Read the model definition and answer for the solid it produces. Units are mm, in the model's axes. Face numbers are marked on the shaded views. A direction names the side the tool comes from. Coordinates: 2 decimals unless noted, no trailing zeros. Order: outer loops, then holes, each group sorted by start corner. A loop starts at its lowest first (then second) coordinate and runs counter-clockwise, first axis right, second up. Notation, with made-up numbers: (-22, -36.5) -> (24, -36.5) arc R18 ccw to (24, -25.5) -> close; hole circle Ø2 at (69, 44). An arc over 180 degrees is marked (long way). Answer as a JSON object with one key per item and string values. Group by question number.
1) Given pin 1 (4 mm diameter, centred on x = 0.5, z = 7, fed in from -Y); pin 2 (1.4 mm diameter, centred on x = 1, z = -7, fed in from +Y); pin 3 (2.5 mm diameter, centred on y = 0, z = 12, fed in from -X), each flat-ended and moving along its own axis, determine where each tip first touches the part or whether it passes through.
2) Section C-C on z = 12 is taken. Count the separate pieces of the cut face and the enclosed holes in it, and give its area (3 significant figures).
3) Section B-B on y = 1.25 is taken. Determine the outline of the cut face in (x, z), and give its area (3 significant figures).
4) Consider L1, parallel to X at y = -8, z = 23.5; L2, parallel to Y at x = -3, z = 9; L3, parallel to Y at x = -4, z = 16. Determine where each line is inside the solid, lowest interval first.
5) Section A-A on x = -6 is taken. Determine the outline of the cut face in (y, z), and give its area (3 significant figures).
6) Determine the mould class of the marked faces 4 and 5 for opening direction X: released by +X, released by -X, zero draft, split by the parting line, or undercut.
7) A tool of negligible diameter and unlimited length cuts with its end or side. For the marked faces 1, 2 and 3, from which of +Z, -Z, +X, -X, +Y, -Y can it reach the whole face along a straight path? Write none if from no direction.
from build123d import *

# Parameters (mm, degrees)
F1_DEPTH = 25


with BuildPart() as f1:
    # F0 (on Top) → F1 (new body, symmetric)
    with BuildSketch(Plane.XY):
        with BuildLine():
            Line((-8.2, 5.5), (-6.56066, 5.5))
            Line((-6.56066, 5.5), (-3.4, 2.33934))
            Line((-3.4, 2.33934), (-3.4, -2.33934))
            Line((-3.4, -2.33934), (-6.56066, -5.5))
            Line((-6.56066, -5.5), (-8.2, -5.5))
            Line((-8.2, -5.5), (-8.2, -2.89))
            Line((-8.2, -2.89), (-8.31, -2.89))
            Line((-8.31, -2.89), (-9.768614, -4.348614))
            ThreePointArc((-9.768614, -4.348614), (-9.939865, -4.604909), (-10, -4.907229))
            Line((-10, -4.907229), (-10, -8.5))
            ThreePointArc((-10, -8.5), (-9.56066, -9.56066), (-8.5, -10))
            Line((-8.5, -10), (-4.907229, -10))
            ThreePointArc((-4.907229, -10), (-4.604909, -9.939865), (-4.348614, -9.768614))
            Line((-4.348614, -9.768614), (-2.89, -8.31))
            Line((-2.89, -8.31), (-2.89, -8.2))
            Line((-2.89, -8.2), (-5.5, -8.2))
            Line((-5.5, -8.2), (-5.5, -6.56066))
            Line((-5.5, -6.56066), (-2.33934, -3.4))
            Line((-2.33934, -3.4), (2.33934, -3.4))
            Line((2.33934, -3.4), (5.5, -6.56066))
            Line((5.5, -6.56066), (5.5, -8.2))
            Line((5.5, -8.2), (2.89, -8.2))
            Line((2.89, -8.2), (2.89, -8.31))
            Line((2.89, -8.31), (4.348614, -9.768614))
            ThreePointArc((4.348614, -9.768614), (4.604909, -9.939865), (4.907229, -10))
            Line((4.907229, -10), (8.5, -10))
            ThreePointArc((8.5, -10), (9.56066, -9.56066), (10, -8.5))
            Line((10, -8.5), (10, -4.907229))
            ThreePointArc((10, -4.907229), (9.939865, -4.604909), (9.768614, -4.348614))
            Line((9.768614, -4.348614), (8.31, -2.89))
            Line((8.31, -2.89), (8.2, -2.89))
            Line((8.2, -2.89), (8.2, -5.5))
            Line((8.2, -5.5), (6.56066, -5.5))
            Line((6.56066, -5.5), (3.4, -2.33934))
            Line((3.4, -2.33934), (3.4, 2.33934))
            Line((3.4, 2.33934), (6.56066, 5.5))
            Line((6.56066, 5.5), (8.2, 5.5))
            Line((8.2, 5.5), (8.2, 2.89))
            Line((8.2, 2.89), (8.31, 2.89))
            Line((8.31, 2.89), (9.768614, 4.348614))
            ThreePointArc((9.768614, 4.348614), (9.939865, 4.604909), (10, 4.907229))
            Line((10, 4.907229), (10, 8.5))
            ThreePointArc((10, 8.5), (9.56066, 9.56066), (8.5, 10))
            Line((8.5, 10), (4.907229, 10))
            ThreePointArc((4.907229, 10), (4.604909, 9.939865), (4.348614, 9.768614))
            Line((4.348614, 9.768614), (2.89, 8.31))
            Line((2.89, 8.31), (2.89, 8.2))
            Line((2.89, 8.2), (5.5, 8.2))
            Line((5.5, 8.2), (5.5, 6.56066))
            Line((5.5, 6.56066), (2.33934, 3.4))
            Line((2.33934, 3.4), (-2.33934, 3.4))
            Line((-2.33934, 3.4), (-5.5, 6.56066))
            Line((-5.5, 6.56066), (-5.5, 8.2))
            Line((-5.5, 8.2), (-2.89, 8.2))
            Line((-2.89, 8.2), (-2.89, 8.31))
            Line((-2.89, 8.31), (-4.348614, 9.768614))
            ThreePointArc((-4.348614, 9.768614), (-4.604909, 9.939865), (-4.907229, 10))
            Line((-4.907229, 10), (-8.5, 10))
            ThreePointArc((-8.5, 10), (-9.56066, 9.56066), (-10, 8.5))
            Line((-10, 8.5), (-10, 4.907229))
            ThreePointArc((-10, 4.907229), (-9.939865, 4.604909), (-9.768614, 4.348614))
            Line((-9.768614, 4.348614), (-8.31, 2.89))
            Line((-8.31, 2.89), (-8.2, 2.89))
            Line((-8.2, 2.89), (-8.2, 5.5))
        make_face()
        Polygon((-7.66, -6.57), (-6.57, -7.66), (-6.57, -8.2), (-8.2, -8.2), (-8.2, -6.57), align=None, mode=Mode.SUBTRACT)
        Polygon((6.57, -7.66), (7.66, -6.57), (8.2, -6.57), (8.2, -8.2), (6.57, -8.2), align=None, mode=Mode.SUBTRACT)
        Polygon((-8.2, 8.2), (-6.57, 8.2), (-6.57, 7.66), (-7.66, 6.57), (-8.2, 6.57), align=None, mode=Mode.SUBTRACT)
        Polygon((7.66, 6.57), (6.57, 7.66), (6.57, 8.2), (8.2, 8.2), (8.2, 6.57), align=None, mode=Mode.SUBTRACT)
    extrude(amount=F1_DEPTH, both=True)


solid = f1.part
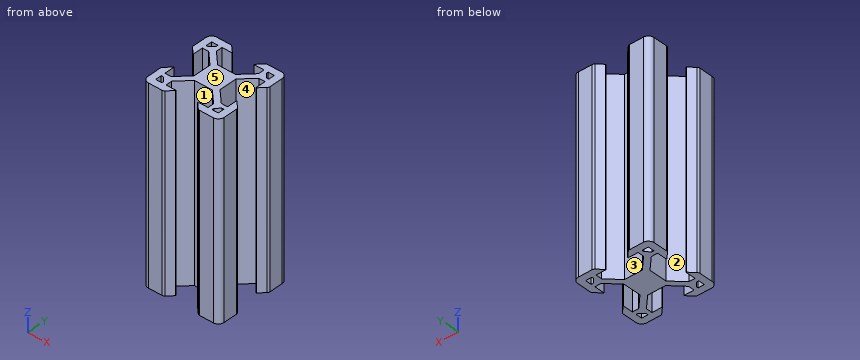
Worked answers:
{
 "1": {"pin 1": "stops at y = -3.56", "pin 2": "stops at y = 3.4", "pin 3": "stops at x = -3.4"},
 "2": {"separate pieces": "1", "enclosed holes": "4", "area": "165 mm²"},
 "3": {"outline": "(-3.4, -25) -> (3.4, -25) -> (3.4, 25) -> (-3.4, 25) -> close", "area": "340 mm²"},
 "4": {"L1": "x = -10 to -8.2, -6.57 to -5.5, 5.5 to 6.57, 8.2 to 10", "L2": "y = -8.42 to -8.2, -4.06 to 4.06, 8.2 to 8.42", "L3": "y = -9.42 to -8.2, -5.06 to -2.94, 2.94 to 5.06, 8.2 to 9.42"},
 "5": {"outline": "(-10, -25) -> (-4.94, -25) -> (-4.94, 25) -> (-10, 25) -> close; (4.94, -25) -> (10, -25) -> (10, 25) -> (4.94, 25) -> close", "area": "506 mm²"},
 "6": {"face 4": "undercut", "face 5": "zero draft"},
 "7": {"face 1": "+Z, -Z, -Y", "face 2": "+Z, -Z", "face 3": "+Z, -Z, +Y"}
}
